Verification items for the finished model (mm, model axes). A direction names the side the tool comes from. Give positions to 0.01 mm unless a question says otherwise; leave off trailing zeros. Loops run counter-clockwise (first coordinate to the right, second up) from the corner with the lowest first, then second, coordinate; pieces in that order, holes last. Notation, with made-up numbers: M -26.5,80 L 8.5,80 A22 cw 8.5,118 Z; hole C 25,85 d11. An arc over 180 degrees is marked long. Answer in a Markdown table with one row per item.
```python
from build123d import *

# Parameters (mm, degrees)
SKETCH1_W            = 60
SKETCH1_H            = 60
BOSS_EXTRUDE1_DEPTH  = 4.2575
SKETCH2_W            = 60
SKETCH2_H            = 60
BOSS_EXTRUDE2_DEPTH  = 1.7425
SKETCH3_W            = 2.095743483
SKETCH3_H            = 23.459092757
CUT_EXTRUDE1_DEPTH   = 4.2575
FILLET1_R            = 1
FILLET2_R            = 5
M3_CLEARANCE_HOLE1_D = 3.2


with BuildPart() as part:
    # Sketch1 → Boss-Extrude1 (new body)
    with BuildSketch(Plane(origin=(0, 0, 0), x_dir=(1, 0, 0), z_dir=(0, 1, 0))):
        Rectangle(SKETCH1_W, SKETCH1_H)
        with BuildLine():
            Line((-9.04644108, -23.573807579), (9.04644108, -23.573807579))
            ThreePointArc((9.04644108, -23.573807579), (14.716185301, 20.518196562), (-25.229791914, 1.01))
            ThreePointArc((-25.229791914, 1.01), (-21.090422846, -13.883679778), (-9.04644108, -23.573807579))
        make_face(mode=Mode.SUBTRACT)
    extrude(amount=BOSS_EXTRUDE1_DEPTH)

    # Sketch2 → Boss-Extrude2 (add)
    with BuildSketch(Plane.XZ):
        Rectangle(SKETCH2_W, SKETCH2_H)
    extrude(amount=BOSS_EXTRUDE2_DEPTH)

    # Sketch3 → Cut-Extrude1 (cut)
    with BuildSketch(Plane(origin=(0, 4.2575, 0), x_dir=(1, 0, 0), z_dir=(0, 1, 0))):
        with Locations((-6.512128259, -34.72527871)):
            Rectangle(SKETCH3_W, SKETCH3_H)
        with Locations((6.512128259, -34.72527871)):
            Rectangle(SKETCH3_W, SKETCH3_H)
    extrude(amount=-CUT_EXTRUDE1_DEPTH, mode=Mode.SUBTRACT)

    # Fillet1
    fillet1_edges = [part.edges().sort_by_distance(p)[0] for p in [
        (-5.464256517, 2.12875, 30),
        (-5.464256517, 2.12875, 23.573807579),
        (-7.56, 2.12875, 30),
        (-7.56, 2.12875, 23.573807579),
        (5.464256517, 2.12875, 30),
        (5.464256517, 2.12875, 23.573807579),
        (7.56, 2.12875, 30),
        (7.56, 2.12875, 23.573807579),
    ]]
    fillet(fillet1_edges, radius=FILLET1_R)

    # Fillet2
    fillet2_edges = [part.edges().sort_by_distance(p)[0] for p in [
        (30, 1.2575, 30),
        (-30, 1.2575, 30),
        (-30, 1.2575, -30),
        (30, 1.2575, -30),
    ]]
    fillet(fillet2_edges, radius=FILLET2_R)

    # M3 Clearance Hole1 (through all)
    with Locations(Plane(origin=(0, -1.7425, 0), x_dir=(-1, 0, 0), z_dir=(0, -1, 0))):
        with Locations((-25, 25), (25, 25), (25, -25), (-25, -25)):
            Hole(M3_CLEARANCE_HOLE1_D / 2)


solid = part.part
```
Item 1: Release check for a two-part mould opening along X. For faces 4 (the flat face through (7.56, 2, 27)), 5 (the cylindrical face through (24.792, 1.3, 23.414)), 6 (the cylindrical face through (-28, 1, -29)), 7 (the flat face through (0, 4.258, 27)) record: released by +X, released by -X, zero draft, split by the parting line, or undercut.
Reported:
| item | result |
|---|---|
| face 4 | undercut |
| face 5 | undercut |
| face 6 | released by -X |
| face 7 | zero draft |
Item 2: Scan lines: L1, parallel to X at y = 2.55, z = 25; L2, parallel to Z at x = 0, y = 2.55; L3, parallel to X at y = 3.3, z = 0. Record each from-to range of solid material in increasing order. Write a range as [from, to].
Reported:
| item | result |
|---|---|
| L1 | x = [-30, -26.6], [-23.4, -7.56], [-5.46, 5.46], [7.56, 23.4], [26.6, 30] |
| L2 | z = [-30, -25.25], [23.57, 30] |
| L3 | x = [-30, -25.25], [25.25, 30] |
Item 3: Go/stop test with flat-tipped pins: pin 1 (4 mm diameter, centred on x = -22.5, z = -5.5, fed in from +Y); pin 2 (1.3 mm diameter, centred on y = 2.5, z = 27, fed in from -X); pin 3 (1.3 mm diameter, centred on y = 2.5, z = 27, fed in from +X). Record where each tip stops, or that it passes through.
Reported:
| item | result |
|---|---|
| pin 1 | stops at y = 0 |
| pin 2 | stops at x = -29.81 |
| pin 3 | stops at x = 29.81 |
Item 4: Sectioned sample at A-A (y = 1.75). State how many separate pieces and enclosed holes the cut face has, and give its area (3 significant figures).
Reported:
| item | result |
|---|---|
| separate pieces | 2 |
| enclosed holes | 4 |
| area | 1,540 mm^2 |
Item 5: Tool access check on faces 1 (the flat face through (-7.56, 2, 27)), 2 (the flat face through (-30, 1, 0)), 3 (the flat face through (0, 2, 23.574)). Record the directions out of +Z, -Z, +X, -X, +Y, -Y that give a thin tool (end or side, any length) a straight path to the whole face; none if there is none.
Reported:
| item | result |
|---|---|
| face 1 | +Z, +Y |
| face 2 | +Z, -Z, -X, +Y, -Y |
| face 3 | +Y |
Item 6: Sectioned sample at C-C (z = 0). Record the cut outline in (x, y), and give its area (3 significant figures).
Reported:
| item | result |
|---|---|
| outline | M -30,-1.74 L 30,-1.74 L 30,4.26 L 25.25,4.26 L 25.25,0 L -25.25,0 L -25.25,4.26 L -30,4.26 Z |
| area | 145 mm^2 |
Item 7: Sectioned sample at B-B (x = 0). Record the cut outline in (y, z), and give its area (3 significant figures).
Reported:
| item | result |
|---|---|
| outline | M -1.74,-30 L 4.26,-30 L 4.26,-25.25 L 0,-25.25 L 0,23.57 L 4.26,23.57 L 4.26,30 L -1.74,30 Z |
| area | 152 mm^2 |
